from build123d import *

# Parameters (mm, degrees)
F1_DEPTH      = 5
F2_R          = 4.99999
F3_R          = 2.5
F4_DEPTH      = 10.001
F4_DEPTH_BACK = 10.001


# Not quite as in the source:
# - a fillet or chamfer is up to 0.001 mm smaller than in the source, because OpenCascade refuses the exact size


with BuildPart() as f1:
    # F0 (on Front) → F1 (new body, symmetric)
    with BuildSketch(Plane.XZ):
        with BuildLine():
            Line((0, -15), (2.5, -15))
            Line((2.5, -15), (2.5, -10.612494996))
            ThreePointArc((2.5, -10.612494996), (3.4861218113, -6.2823679771), (6.25, -2.806247498))
            ThreePointArc((6.25, -2.806247498), (9.0138781887, 0.6698729811), (10, 5))
            Line((10, 5), (10, 15))
            Line((10, 15), (5, 15))
            Line((5, 15), (5, 5))
            ThreePointArc((5, 5), (3.5355339059, 1.4644660941), (0, 0))
            ThreePointArc((0, 0), (-3.5355339059, 1.4644660941), (-5, 5))
            Line((-5, 5), (-5, 15))
            Line((-5, 15), (-10, 15))
            Line((-10, 15), (-10, 5))
            ThreePointArc((-10, 5), (-9.0138781887, 0.6698729811), (-6.25, -2.806247498))
            ThreePointArc((-6.25, -2.806247498), (-3.4861218113, -6.2823679771), (-2.5, -10.612494996))
            Line((-2.5, -10.612494996), (-2.5, -15))
            Line((-2.5, -15), (0, -15))
        make_face()
    extrude(amount=F1_DEPTH, both=True)

    # F2 (radius 5 in the source; OpenCascade refuses exactly that, so slightly less here)
    f2_edges = [f1.edges().sort_by_distance(p)[0] for p in [
        (-7.5, -5, 15),
        (7.5, -5, 15),
        (7.5, 5, 15),
        (-7.5, 5, 15),
    ]]
    fillet(f2_edges, radius=F2_R)

    # F3 (on Right) → F4 (cut, two sides)
    with BuildSketch(Plane.YZ) as f4_sk:
        with Locations((0, 10)):
            Circle(F3_R)
    extrude(amount=-F4_DEPTH, mode=Mode.SUBTRACT)
    extrude(f4_sk.sketch, amount=F4_DEPTH_BACK, mode=Mode.SUBTRACT)


solid = f1.part
CAD build for the part. Positions are in the model's coordinates, mm. A direction names the side the tool comes from. Round coordinates to 2 decimals unless told otherwise and drop trailing zeros. Order: outer loops, then holes, each group sorted by start corner. A loop starts at its lowest first (then second) coordinate and runs counter-clockwise, first axis right, second up. Notation, with made-up numbers: (62, 47) -> (120, 47) arc R21 ccw to (120, 75) -> close; hole circle Ø2 at (-0.5, -31.5). An arc over 180 degrees is marked (long way). Write each question's results on one line, items separated by ' | '.
1. Cut at D-D (y = 3.5). Give the cut face in (x, z), plus the area to 3 significant figures.
Findings below:
outline: (-10, 5) arc R10 ccw to (-6.25, -2.81) arc R10 cw to (-2.5, -10.61) -> (-2.5, -15) -> (2.5, -15) -> (2.5, -10.61) arc R10 cw to (6.25, -2.81) arc R10 ccw to (10, 5) -> (10, 13.57) -> (5, 13.57) -> (5, 5) arc R5 cw to (-5, 5) -> (-5, 13.57) -> (-10, 13.57) -> close | area: 264 mm²
2. Cut at B-B (y = 0.5). Give the cut face in (x, z), plus the area to 3 significant figures.
Findings below:
outline: (-10, 5) arc R10 ccw to (-6.25, -2.81) arc R10 cw to (-2.5, -10.61) -> (-2.5, -15) -> (2.5, -15) -> (2.5, -10.61) arc R10 cw to (6.25, -2.81) arc R10 ccw to (10, 5) -> (10, 7.55) -> (5, 7.55) -> (5, 5) arc R5 cw to (-5, 5) -> (-5, 7.55) -> (-10, 7.55) -> close; (-10, 12.45) -> (-5, 12.45) -> (-5, 14.97) -> (-10, 14.97) -> close; (5, 12.45) -> (10, 12.45) -> (10, 14.97) -> (5, 14.97) -> close | area: 229 mm²
3. Cut at A-A (z = 13). Give the cut face in (x, y).
Findings below:
outline: (-10, -4) -> (-5, -4) -> (-5, 4) -> (-10, 4) -> close; (5, -4) -> (10, -4) -> (10, 4) -> (5, 4) -> close
4. Pull direction X, two halves, no side cores. Call faces 1 (the face through (-2.5, 0, -13)), 2 (the face through (5, 0, 7)), 3 (the face through (0, 5, -2)): pulls with the +X half, pulls with the -X half, needs draft (parallel to the pull), parting line crosses it, or undercut.
Findings below:
face 1: pulls with the -X half | face 2: undercut | face 3: needs draft
5. 3-axis set-ups, long thin cutter, end or side, ignore diameter. For faces 4 (the face through (2.5, 0, -13)), 5 (the face through (-5, 2, 8)), 6 (the face through (0, 0, -15)): which of +Z, -Z, +X, -X, +Y, -Y reach the whole face in a straight line?
Findings below:
face 4: -Z, +X, +Y, -Y | face 5: +Z, +Y, -Y | face 6: -Z, +X, -X, +Y, -Y
6. Flat gauge pins, fed straight in: P1, Ø5, axis at y = 1, z = -12, coming from the +X side; P2, Ø1.5, axis at y = 2.5, z = -6, coming from the +X side; P3, Ø3, axis at x = 2.5, y = -0.5, coming from the +Z side. Where does each tip first touch, or does it go through?
Findings below:
P1: stops at x = 2.56 | P2: stops at x = 4.06 | P3: stops at z = 2
7. Wall check: line 1 along X through (y, z) = (-2.25, 6.5); line 2 along Y through (x, z) = (7.2, 10); line 3 along X through (y, z) = (-2.5, -12.25). Give the ranges that are in metal, low to high. Write a range as [from, to].
Findings below:
line 1: x = [-10, -5], [5, 10] | line 2: y = [-5, -2.5], [2.5, 5] | line 3: x = [-2.5, 2.5]
